from build123d import *

# Parameters (mm, degrees)
SKIZZE2_W                       = 15
SKIZZE2_H                       = 7
AUFSATZ_LINEAR_AUSTRAGEN1_DEPTH = 1
SKIZZE3_R                       = 2.25
SKIZZE3_R_2                     = 1
AUFSATZ_LINEAR_AUSTRAGEN2_DEPTH = 15
SCHNITT_LINEAR_START            = -5
SCHNITT_LINEAR_AUSTRAGEN1_DEPTH = 5
SKIZZE7_W                       = 5.129171307
SKIZZE7_H                       = 1
AUFSATZ_LINEAR_AUSTRAGEN3_DEPTH = 2.5
FASE1_SIZE                      = 0.5
VERST_RKUNGSFASE_DEPTH          = 5
AUFSATZ_LINEAR_AUSTRAGEN5_DEPTH = 5


with BuildPart() as part:
    # Skizze2 → Aufsatz-Linear austragen1 (new body)
    with BuildSketch(Plane(origin=(0, 0, 0), x_dir=(1, 0, 0), z_dir=(0, 1, 0))):
        Rectangle(SKIZZE2_W, SKIZZE2_H)
    extrude(amount=AUFSATZ_LINEAR_AUSTRAGEN1_DEPTH)

    # Skizze3 → Aufsatz-Linear austragen2 (add)
    with BuildSketch(Plane(origin=(7.5, 0, 0), x_dir=(0, 0, -1), z_dir=(1, 0, 0))):
        with Locations((-3.5, 2.25)):
            Circle(SKIZZE3_R)
        with Locations((-3.5, 2.25)):
            Circle(SKIZZE3_R_2, mode=Mode.SUBTRACT)
    extrude(amount=-AUFSATZ_LINEAR_AUSTRAGEN2_DEPTH)

    # Skizze5 → Schnitt-Linear austragen1 (cut)
    with BuildSketch(Plane(origin=(7.5, 0, 0), x_dir=(0, 0, -1), z_dir=(1, 0, 0)).offset(SCHNITT_LINEAR_START)):
        with BuildLine():
            Line((-1.629171307, 1), (-1.629171307, 0))
            Line((-1.629171307, 0), (-3.5, 0))
            ThreePointArc((-3.5, 0), (-4.560660172, 4.234313483), (-1.629171307, 1))
        make_face()
    extrude(amount=-SCHNITT_LINEAR_AUSTRAGEN1_DEPTH, mode=Mode.SUBTRACT)

    # Skizze7 → Aufsatz-Linear austragen3 (add)
    with BuildSketch(Plane(origin=(7.5, 0, 0), x_dir=(0, 0, -1), z_dir=(1, 0, 0))):
        with Locations((0.935414346, 0.5)):
            Rectangle(SKIZZE7_W, SKIZZE7_H)
    aufsatz_linear_austragen3 = extrude(amount=AUFSATZ_LINEAR_AUSTRAGEN3_DEPTH)

    # Spiegeln1: Aufsatz-Linear austragen3 across plane
    add(aufsatz_linear_austragen3.mirror(Plane(origin=(0, 0, 0), x_dir=(0, 0, 1), z_dir=(1, 0, 0))))

    # Fase1
    fase1_edges = [part.edges().sort_by_distance(p)[0] for p in [
        (-7.5, 2.25, 4.5),
        (7.5, 2.25, 4.5),
        (2.5, 2.25, 4.5),
        (-2.5, 2.25, 4.5),
    ]]
    chamfer(fase1_edges, length=FASE1_SIZE)

    # Skizze8 → Verstärkungsfase (add)
    with BuildSketch(Plane(origin=(7.5, 0, 0), x_dir=(0, 0, -1), z_dir=(1, 0, 0))):
        Polygon((-1.629171307, 1), (3.5, 1), (-2.423928807, 4.225998681), align=None)
    extrude(amount=-VERST_RKUNGSFASE_DEPTH)

    # Skizze9 → Aufsatz-Linear austragen5 (add)
    with BuildSketch(Plane.ZY.offset(7.5)):
        Polygon((1.629171307, 1), (-3.5, 1), (2.423928807, 4.225998681), align=None)
    extrude(amount=-AUFSATZ_LINEAR_AUSTRAGEN5_DEPTH)


solid = part.part
Model file for the job. Use its own axes, mm. A direction names the side the tool comes from. Give positions to 0.01 mm unless a question says otherwise; leave off trailing zeros. Loops run counter-clockwise (first coordinate to the right, second up) from the corner with the lowest first, then second, coordinate; pieces in that order, holes last. Notation, with made-up numbers: (3.25, 48) -> (35.25, 48) arc R18 cw to (35.25, 76) -> close; hole circle Ø6 at (-27, -18.5). An arc over 180 degrees is marked (long way). Use a Markdown table: item, result. Add a question column.
(1) Slice it at A-A on y = 2.25. List the corners of the cut face in (x, z), and give its area (3 significant figures).
(2) Tool access for faces 1 (the flat face through (-9, 1, -1)), 2 (the flat face through (5.04, 2.59, -0.58)), 3 (the cylindrical face through (-5, 2.3, 4.5)), 4 (the flat face through (8.7, 0.5, 1.629)), 5 (the flat face through (2.5, 2, 1)): list every direction of +Z, -Z, +X, -X, +Y, -Y with a clear straight run to the whole face (end or side of a thin tool).
(3) Drop flat-ended pins along their axis: pin 1 Ø0.8 at (x, y) = (0.5, 0.5) entering from +Z; pin 2 Ø2 at (y, z) = (1.5, 3) entering from -X; pin 3 Ø0.8 at (x, z) = (8.5, -0.5) entering from +Y. Give the stop position or say it passes through.
(4) Mould opens along X. For faces 6 (the flat face through (-10, 0.5, -0.9)), 7 (the flat face through (0, 1, -1)), 8 (the flat face through (10, 0.5, -0.9)) say: +X half, -X half, draft (parallel to the pull), parting line (faces both ways), or undercut.
(5) Slice it at B-B on x = 3.25. List the corners of the cut face in (y, z).
(6) Wall check: line 1 along X through (y, z) = (2.6, 0.25); line 2 along Y through (x, z) = (-4.3, 3.5); line 3 along Z through (x, y) = (-6, 2.75). Give the ranges that are in metal, low to high.
(7) Slice it at D-D on z = 2.75. Give the number of separate pieces and of enclosed holes in the cut face, and give its area (3 significant figures).
(8) Slice it at C-C on z = -1.25. List the corners of the cut face in (x, y), and give its area (3 significant figures).
Filled sheet:
| question | item | result |
|---|---|---|
| 1 | outline | (-7.5, -1.2) -> (-2.5, -1.2) -> (-2.5, 2) -> (-3, 2.5) -> (-7, 2.5) -> (-7.5, 2) -> close; (-7.5, 5) -> (-7, 4.5) -> (-3, 4.5) -> (-2.5, 5) -> (-2.5, 5.75) -> (-7.5, 5.75) -> close; (2.5, -1.2) -> (7.5, -1.2) -> (7.5, 2) -> (7, 2.5) -> (3, 2.5) -> (2.5, 2) -> close; (2.5, 5) -> (3, 4.5) -> (7, 4.5) -> (7.5, 5) -> (7.5, 5.75) -> (2.5, 5.75) -> close |
| 1 | area | 48.5 mm2 |
| 2 | face 1 | +Z, -Z, -X, +Y |
| 2 | face 2 | -Z, +X, -X, +Y |
| 2 | face 3 | +X, -X |
| 2 | face 4 | +Z, +X, +Y, -Y |
| 2 | face 5 | +Z, +Y |
| 3 | pin 1 | z = 1.63 |
| 3 | pin 2 | x = -7.5 |
| 3 | pin 3 | y = 1 |
| 4 | face 6 | -X half |
| 4 | face 7 | undercut |
| 4 | face 8 | +X half |
| 5 | outline | (0, -3.5) -> (1, -3.5) -> (4.23, 2.42) arc R2.25 ccw (long way) to (0, 3.5) -> close; hole circle Ø2 at (2.25, 3.5) |
| 6 | line 1 | -7.5 to -2.5, 2.5 to 7.5 |
| 6 | line 2 | 0 to 1.25, 3.25 to 4.5 |
| 6 | line 3 | -0.29 to 2.63, 4.37 to 5.69 |
| 7 | separate pieces | 4 |
| 7 | enclosed holes | 0 |
| 7 | area | 29.2 mm2 |
| 8 | outline | (-10, 0) -> (10, 0) -> (10, 1) -> (7.5, 1) -> (7.5, 2.23) -> (2.5, 2.23) -> (2.5, 1) -> (-2.5, 1) -> (-2.5, 2.23) -> (-7.5, 2.23) -> (-7.5, 1) -> (-10, 1) -> close |
| 8 | area | 32.3 mm2 |
